The drawing under review shows one solid part. Ordinate dimensions are in mm from its lowest x, y, z. Round coordinates to 2 decimals unless told otherwise and drop trailing zeros. Order: outer loops, then holes, each group sorted by start corner. A loop starts at its lowest first (then second) coordinate and runs counter-clockwise, first axis right, second up.
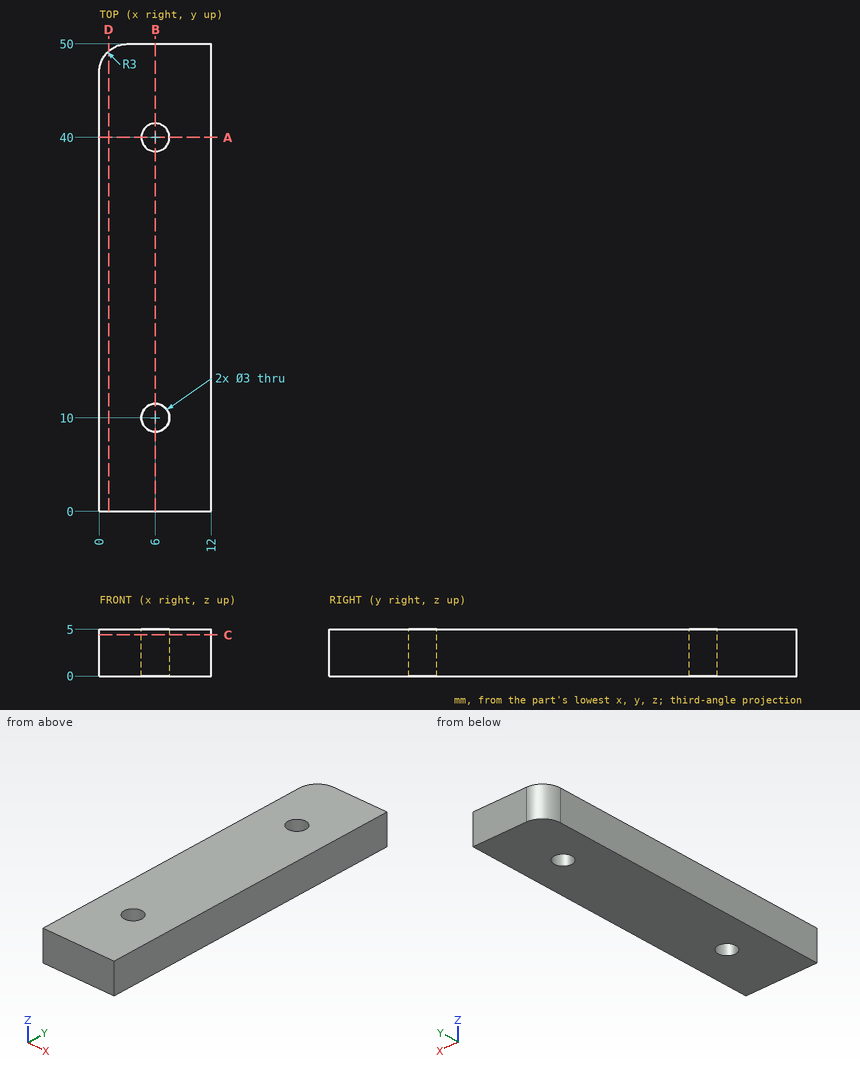
Q1. Take a section at A-A, the plane y = 40. State the section outline as (x, z) points, plus the area to 3 significant figures.
Q2. Take a section at B-B, the plane x = 6. State the section outline as (y, z) points, plus the area to 3 significant figures.
Q3. Take a section at D-D, the plane x = 1. State the section outline as (y, z) points.
Q4. Take a section at C-C, the plane z = 4.4. State the section outline as (x, y) points.
Q5. Wall thickness on line 1 (Y direction, x = 6, z = 2.8); line 2 (X direction, y = 10, z = 2.25); line 3 (Y direction, x = 5.25, z = 3.25): over which ranges is each line inside the solid? List them lowest first.
Q6. Clearance check with a flat-ended pin moving along its axis: pin 1 (3.5 mm diameter, centred on x = 6, y = 40, fed in from +Z). State where the tip first meets the part, or that it passes through.
Working result:
1. outline: (0, 0) - (4.5, 0) - (4.5, 5) - (0, 5) - close; (7.5, 0) - (12, 0) - (12, 5) - (7.5, 5) - close
1. area: 45.0 mm2
2. outline: (0, 0) - (8.5, 0) - (8.5, 5) - (0, 5) - close; (11.5, 0) - (38.5, 0) - (38.5, 5) - (11.5, 5) - close; (41.5, 0) - (50, 0) - (50, 5) - (41.5, 5) - close
2. area: 220 mm2
3. outline: (0, 0) - (49.24, 0) - (49.24, 5) - (0, 5) - close
4. outline: (0, 0) - (12, 0) - (12, 50) - (3, 50) arc R3 ccw to (0, 47) - close; hole circle Ø3 at (6, 10); hole circle Ø3 at (6, 40)
5. line 1: y = 0 to 8.5, 11.5 to 38.5, 41.5 to 50
5. line 2: x = 0 to 4.5, 7.5 to 12
5. line 3: y = 0 to 8.7, 11.3 to 38.7, 41.3 to 50
6. pin 1: stops at z = 5
